```python
from build123d import *

# Parameters (mm, degrees)
SKETCH_1_W      = 35.318125
SKETCH_1_H      = 30
SKETCH_1_R      = 0.8
SKETCH_1_W_2    = 4
SKETCH_1_H_2    = 20
EXTRUDE_1_DEPTH = 1.6
FILLET_1_R      = 2


with BuildPart() as part:
    # 草图1 → 凸台-拉伸1 (new body)
    with BuildSketch(Plane.XY):
        with Locations((19.3409375, -3.5)):
            Rectangle(SKETCH_1_W, SKETCH_1_H)
        with Locations((14.38454248, 3.5)):
            Circle(SKETCH_1_R, mode=Mode.SUBTRACT)
        with Locations((24.38454248, 3.5)):
            Circle(SKETCH_1_R, mode=Mode.SUBTRACT)
        with Locations((6.681875, -3.5)):
            Rectangle(SKETCH_1_W_2, SKETCH_1_H_2, mode=Mode.SUBTRACT)
        with Locations((32, -3.5)):
            Rectangle(SKETCH_1_W_2, SKETCH_1_H_2, mode=Mode.SUBTRACT)
    extrude(amount=EXTRUDE_1_DEPTH)

    # 圆角1
    fillet_1_edges = [part.edges().sort_by_distance(p)[0] for p in [
        (1.681875, 11.5, 0.8),
        (37, 11.5, 0.8),
        (37, -18.5, 0.8),
        (1.681875, -18.5, 0.8),
    ]]
    fillet(fillet_1_edges, radius=FILLET_1_R)


solid = part.part
```
Could you check a few things on this model? Use its own coordinates, in mm. A direction names the side the tool comes from. Coordinates: 2 decimals unless noted, no trailing zeros. Loops run counter-clockwise (first coordinate to the right, second up) from the corner with the lowest first, then second, coordinate; pieces in that order, holes last. Notation, with made-up numbers: M 25.25,24.25 L 72.25,24.25 A19 ccw 72.25,58.25 Z; hole C 87.5,26.25 d7. An arc over 180 degrees is marked long. Put each result on its own line as item: value. Start each with the question number.
(1) Suppose I cut it at A-A on x = 6. Please give me the cut outline in (y, z).
(2) Suppose I cut it at C-C on z = 0.65. Please give me the cut outline in (x, y), then the cut area to 3 significant figures.
(3) Will this pin go through, and if not, where does the flat tip stop? P1, Ø10, axis at x = 16.5, y = 0.5, coming from the -Z side.
(4) For faces 4 (the face through (36.4, -17.93, 0.81)), 5 (the face through (7, -13.5, 1)), which set-ups out of +Z, -Z, +X, -X, +Y, -Y let a thin tool reach every point of the face, with its end or its side?
(5) Suppose I cut it at B-B on y = 3.5. Please give me the cut outline in (x, z).
(6) I need wall thicknesses on line 1 (X direction, y = 6.25, z = 1.15); line 2 (Y direction, x = 6.5, z = 1.1); line 3 (Y direction, x = 3, z = 0.7). Which ranges of each line are inside material? Lowest first, please. Write a range as from..to.
(7) Thinking about a two-plate mould opening in Y: for faces 1 (the face through (32, -13.5, 1)), 2 (the face through (19, -3, 1.6)), 3 (the face through (19, 11.5, 1)), which applies, pulls with the +Y half, pulls with the -Y half, needs draft (parallel to the pull), parting line crosses it, or undercut?
Solutions:
1. outline: M -18.5,0 L -13.5,0 L -13.5,1.6 L -18.5,1.6 Z; M 6.5,0 L 11.5,0 L 11.5,1.6 L 6.5,1.6 Z
2. outline: M 1.68,-16.5 A2 ccw 3.68,-18.5 L 35,-18.5 A2 ccw 37,-16.5 L 37,9.5 A2 ccw 35,11.5 L 3.68,11.5 A2 ccw 1.68,9.5 Z; hole M 4.68,-13.5 L 8.68,-13.5 L 8.68,6.5 L 4.68,6.5 Z; hole C 14.38,3.5 d1.6; hole C 24.38,3.5 d1.6; hole M 30,-13.5 L 34,-13.5 L 34,6.5 L 30,6.5 Z
2. area: 892 mm2
3. P1: stops at z = 0
4. face 4: +Z, -Z, +X, -Y
4. face 5: +Z, -Z
5. outline: M 1.68,0 L 4.68,0 L 4.68,1.6 L 1.68,1.6 Z; M 8.68,0 L 13.58,0 L 13.58,1.6 L 8.68,1.6 Z; M 15.18,0 L 23.58,0 L 23.58,1.6 L 15.18,1.6 Z; M 25.18,0 L 30,0 L 30,1.6 L 25.18,1.6 Z; M 34,0 L 37,0 L 37,1.6 L 34,1.6 Z
6. line 1: x = 1.68..4.68, 8.68..30, 34..37
6. line 2: y = -18.5..-13.5, 6.5..11.5
6. line 3: y = -18.38..11.38
7. face 1: undercut
7. face 2: needs draft
7. face 3: pulls with the +Y half
